Autodesk Inventor part; units mm, degrees
ref_plane "YZ Plane" through (0, 0, 0) normal (1, 0, 0) x (0, 1, 0)
ref_plane "XZ Plane" through (0, 0, 0) normal (0, 1, 0) x (-1, 0, 0)
ref_plane "XY Plane" through (0, 0, 0) normal (0, 0, 1) x (1, 0, 0)
sketch "Sketch1" plane through (0, 0, 0) normal (0, 0, 1) x (1, 0, 0)
  line L0 (-45, 10) -> (45, 10)
  line L1 (45, 10) -> (45, -10)
  line L2 (45, -10) -> (-45, -10)
  line L3 (-45, -10) -> (-45, 10)
  point P0 (0, 0)
  point P1 (0, 10)
  point P2 (-45, 0)
  dimension "d0" = 20
  dimension "d1" = 90
extrude "Extrusion1" add sketch "Sketch1" along normal blind 13
sketch "Sketch3" plane through (-45, 10, 0) normal (0, 1, 0) x (1, 0, 0)
  line L0 (90, 0) -> (90, -13)
  line L1 (90, -13) -> (0, -13)
  line L2 (90, -13) -> (60.5, -13)
  line L3 (60.5, -13) -> (60.5, -7)
  line L4 (60.5, -7) -> (90, -7)
  line L5 (90, -7) -> (90, -13)
  point P0 (45, 0)
  point P1 (60.5, -13)
  dimension "d8" = 6
  dimension "d20" = 15.5
extrude "Extrusion2" cut sketch "Sketch3" against normal through all
mirror "Mirror1" about plane through (0, 0, 0) normal (1, 0, 0) of "Extrusion2"
sketch "Sketch4" plane through (-45, 10, 0) normal (0, 1, 0) x (1, 0, 0)
  line L0 (42, -26.343) -> (42, -14.343)
  line L1 (48, -22.843) -> (48, -17.843)
  line L2 (45, -24.843) -> (45, -15.843)
  line L3 (39, -27.343) -> (39, -13.343)
  line L4 (8, -14.343) -> (8, -26.343)
  line L5 (11, -13.343) -> (11, -27.343)
  line L6 (5, -15.843) -> (5, -24.843)
  line L7 (2, -17.843) -> (2, -22.843)
  circle A0 centre (45, -23.343) radius 15.65
  line L8 (90, 0) -> (0, 0)
  point P0 (45, 0)
  point P1 (45, 0)
  dimension "d21" = 31.3
  dimension "d22" = 23.343
extrude "Extrusion3" cut sketch "Sketch4" against normal through all
chamfer "Chamfer1" distance 1 distance2 3 1 edges at (-15.5, 0, 13) measured on face at (-12.9967, 3.3333, 13)
chamfer "Chamfer2" distance 1 distance2 3 1 edges at (15.5, 0, 13) measured on face at (14.2483, -3.3333, 13)
sketch "Sketch5" plane through (0, 0, 0) normal (0, 0, -1) x (-1, 0, 0)
  line L0 (45, -10) -> (-45, -10)
  line L1 (0, 23.0048) -> (0, -23.0048) construction
  point P0 (0, 0)
  point P1 (-35, 0)
  point P2 (35, 0)
  point P3 (0, 0)
  dimension "d23" = 70
hole "Hole1" at (35, 0, 0) at (-35, 0, 0) direction (0, 0, 1) diameter 5 end through all
sketch "Sketch6" plane through (-45, 10, 0) normal (0, 1, 0) x (1, 0, 0)
  line L0 (60.5, -10) -> (59.5, -13)
  line L1 (60.5, -10) -> (60.5, -7)
  line L2 (60.5, -7) -> (90, -7)
  line L3 (90, 0) -> (90, -7)
  line L4 (90, 0) -> (0, 0)
  line L5 (0, 0) -> (0, -7)
  line L6 (0, -7) -> (29.5, -7)
  line L7 (29.5, -7) -> (29.5, -10)
  line L8 (30.5, -13) -> (29.5, -10)
  line L9 (33.255, -13) -> (30.5, -13)
  arc A0 (56.745, -13) -> (33.255, -13) centre (45, -23.343) ccw
  line L10 (59.5, -13) -> (56.745, -13)
  line L11 (60.5, -7) -> (60.5, 0)
  line L12 (90, 0) -> (0, 0)
  line L13 (29.5, -7) -> (29.5, 0)
  line L14 (0, 0) -> (90, 0)
  point P0 (45, 0)
extrude "Extrusion4" add sketch "Sketch6" along normal blind 10
sketch "Sketch7" plane through (-45, -10, 7) normal (0, 0, 1) x (1, 0, 0)
  line L0 (29.5, 23.5) -> (60.5, 23.5)
  line L1 (60.5, 23.5) -> (60.5, 20)
  line L2 (60.5, 20) -> (29.5, 20)
  line L3 (29.5, 20) -> (29.5, 23.5)
  line L4 (13, 20) -> (27.9, 20)
  line L5 (90, 30) -> (0, 30)
  line L6 (60.5, 30) -> (60.5, 0)
  point P0 (45, 10)
  point P1 (45, 23.5)
  point P2 (45, 30)
  dimension "d33" = 3.5
extrude "Extrusion5" cut sketch "Sketch7" against normal through all both and the other way through all
properties part number "0008-10-004 Fixare seringa" material "ABS Plastic"
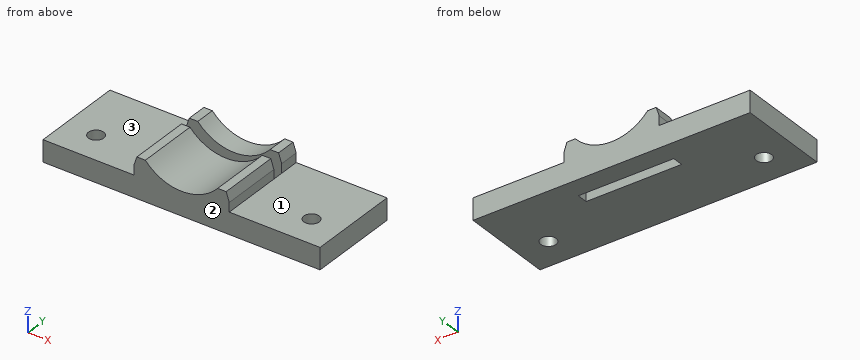
Part model, mm, in its own coordinate system. Face numbers are marked on the shaded views. A direction names the side the tool comes from. Give positions to 0.01 mm unless a question says otherwise; leave off trailing zeros. Loops run counter-clockwise (first coordinate to the right, second up) from the corner with the lowest first, then second, coordinate; pieces in that order, holes last. Notation, with made-up numbers: M 68,0 L 124,0 A17 ccw 124,5 Z; hole C -10.75,-34 d1. An arc over 180 degrees is marked long. Put each result on its own line as item: value. Start each with the question number.
1) 3-axis set-ups, long thin cutter, end or side, ignore diameter. For the marked faces 1, 2 and 3: which of +Z, -Z, +X, -X, +Y, -Y reach the whole face in a straight line?
2) Saw through at B-B (x = 35). List the corners of the cut face in (y, z).
3) Probe probe 1 along X at (y, z) = (0, 2); probe 2 along Y at (x, z) = (-10.5, 7.25); probe 3 along Y at (x, z) = (35, 3.25). List the from-to ranges inside material, lowest first.
4) Saw through at C-C (z = 5.5). List the corners of the cut face in (x, y).
5) Saw through at D-D (z = 11.5). List the corners of the cut face in (x, y), then the cut area to 3 significant figures.
6) Saw through at A-A (y = 0). List the corners of the cut face in (x, z) (3 decimals).
7) Flat gauge pins, fed straight in: pin 1 (6 mm diameter, centred on y = 2.5, z = 8.5, fed in from +X); pin 2 (0.9 mm diameter, centred on y = -5, z = 9, fed in from +X); pin 3 (6.5 mm diameter, centred on x = -35, y = 0, fed in from +Z); pin 4 (1.5 mm diameter, centred on y = 8.5, z = 11, fed in from +X). Where does each tip first touch, or does it go through?
Numbers:
1. face 1: +Z, +X, +Y, -Y
1. face 2: +Z, -Z, +X, -X, -Y
1. face 3: +Z, -X, +Y, -Y
2. outline: M -10,0 L -2.5,0 L -2.5,7 L -10,7 Z; M 2.5,0 L 20,0 L 20,7 L 2.5,7 Z
3. probe 1: -45 to -37.5, -32.5 to 32.5, 37.5 to 45
3. probe 2: -10 to 10, 13.5 to 20
3. probe 3: -10 to -2.5, 2.5 to 20
4. outline: M -45,-10 L 45,-10 L 45,20 L -45,20 Z; hole C -35,0 d5; hole M -15.5,10 L 15.5,10 L 15.5,13.5 L -15.5,13.5 Z; hole C 35,0 d5
5. outline: M -15,-10 L -10.23,-10 L -10.23,10 L -15,10 Z; M -15,13.5 L -10.23,13.5 L -10.23,20 L -15,20 Z; M 10.23,-10 L 15,-10 L 15,10 L 10.23,10 Z; M 10.23,13.5 L 15,13.5 L 15,20 L 10.23,20 Z
5. area: 253 mm^2
6. outline: M -45,0 L -37.5,0 L -37.5,7 L -45,7 Z; M -32.5,0 L 32.5,0 L 32.5,7 L 15.5,7 L 15.5,10 L 14.5,13 L 11.745,13 A15.65 cw -11.745,13 L -14.5,13 L -15.5,10 L -15.5,7 L -32.5,7 Z; M 37.5,0 L 45,0 L 45,7 L 37.5,7 Z
7. pin 1: x = 45
7. pin 2: x = 15.5
7. pin 3: z = 7
7. pin 4: x = 15.42
